```python
from build123d import *

# Parameters (mm, degrees)
SKETCH1_W                               = 16
SKETCH1_H                               = 16
BASE_DEPTH                              = 45
SKETCH3_R                               = 8
SLOTFORANOTHERPART_DEPTH                = 9
CHAMFERFORSLOT_DEPTH                    = 9
M5X0_8_TAPPED_HOLE_FOR_SLOTSCREW_D      = 4.2
M5X0_8_TAPPED_HOLE_FOR_SLOTSCREW_DEPTH  = 11.1381927
M5X0_8_TAPPED_HOLE_FOR_SLOTSCREW_TIP    = 1.2618073
M3X0_5_TAPPED_HOLE_FOR_ROD_FIXING_D     = 2.5
M3X0_5_TAPPED_HOLE_FOR_ROD_FIXING_DEPTH = 6.748924226
M3X0_5_TAPPED_HOLE_FOR_ROD_FIXING_TIP   = 0.751075774
F_10_2_10_2_ROD_HOLE_D                  = 10.2
F_10_2_10_2_ROD_HOLE_DEPTH              = 11.935610843
F_10_2_10_2_ROD_HOLE_CSINK_D            = 11
F_10_2_10_2_ROD_HOLE_CSINK_ANGLE        = 90
F_10_2_10_2_ROD_HOLE_TIP                = 3.064389157


with BuildPart() as part:
    # Sketch1 → Base (new body)
    with BuildSketch(Plane.XY):
        Rectangle(SKETCH1_W, SKETCH1_H)
    extrude(amount=BASE_DEPTH)

    # Sketch3 → SlotForAnotherPart (cut, through all)
    with BuildSketch(Plane(origin=(0, 0, 0), x_dir=(0, 0, -1), z_dir=(1, 0, 0))):
        with BuildLine():
            Line((-8.000000039, 8), (-18, 8))
            Line((-18, 8), (-18, -8))
            Line((-18, -8), (-8, -8))
            ThreePointArc((-8, -8), (-16, -1.9e-08), (-8.000000039, 8))
        make_face()
        with Locations((-8, 0)):
            Circle(SKETCH3_R)
        with BuildLine():
            Line((1.927362357, 8), (-8.000000039, 8))
            ThreePointArc((-8.000000039, 8), (-2.343145764, 5.656854263), (0, 0))
            ThreePointArc((0, 0), (-2.343145751, -5.656854249), (-8, -8))
            Line((-8, -8), (1.927362357, -8))
            Line((1.927362357, -8), (1.927362357, 8))
        make_face()
    extrude(amount=-SLOTFORANOTHERPART_DEPTH, mode=Mode.SUBTRACT)

    # Sketch3_3 → ChamferForSlot (cut, through all)
    with BuildSketch(Plane(origin=(0, 0, 0), x_dir=(0, 0, -1), z_dir=(1, 0, 0))):
        with BuildLine():
            Line((1.927362357, 8), (-8.000000039, 8))
            ThreePointArc((-8.000000039, 8), (-2.343145764, 5.656854263), (0, 0))
            ThreePointArc((0, 0), (-2.343145751, -5.656854249), (-8, -8))
            Line((-8, -8), (1.927362357, -8))
            Line((1.927362357, -8), (1.927362357, 8))
        make_face()
    extrude(amount=CHAMFERFORSLOT_DEPTH, mode=Mode.SUBTRACT)

    # M5x0.8 Tapped Hole for SlotScrew
    with Locations(Plane(origin=(8, 0, 0), x_dir=(0, 0, -1), z_dir=(1, 0, 0))):
        with Locations((-8, 0)):
            Hole(M5X0_8_TAPPED_HOLE_FOR_SLOTSCREW_D / 2, depth=M5X0_8_TAPPED_HOLE_FOR_SLOTSCREW_DEPTH)
            with Locations((0, 0, -(M5X0_8_TAPPED_HOLE_FOR_SLOTSCREW_DEPTH + M5X0_8_TAPPED_HOLE_FOR_SLOTSCREW_TIP / 2))):  # 118° drill point
                Cone(0, M5X0_8_TAPPED_HOLE_FOR_SLOTSCREW_D / 2, M5X0_8_TAPPED_HOLE_FOR_SLOTSCREW_TIP, mode=Mode.SUBTRACT)

    # M3x0.5 Tapped Hole for Rod Fixing
    with Locations(Plane(origin=(8, 0, 0), x_dir=(0, 0, -1), z_dir=(1, 0, 0))):
        with Locations((-40, 0)):
            Hole(M3X0_5_TAPPED_HOLE_FOR_ROD_FIXING_D / 2, depth=M3X0_5_TAPPED_HOLE_FOR_ROD_FIXING_DEPTH)
            with Locations((0, 0, -(M3X0_5_TAPPED_HOLE_FOR_ROD_FIXING_DEPTH + M3X0_5_TAPPED_HOLE_FOR_ROD_FIXING_TIP / 2))):  # 118° drill point
                Cone(0, M3X0_5_TAPPED_HOLE_FOR_ROD_FIXING_D / 2, M3X0_5_TAPPED_HOLE_FOR_ROD_FIXING_TIP, mode=Mode.SUBTRACT)

    # 10.2 _10.2_ Rod Hole
    with Locations(Plane.XY.offset(45)):
        with Locations((0, 0)):
            CounterSinkHole(F_10_2_10_2_ROD_HOLE_D / 2, F_10_2_10_2_ROD_HOLE_CSINK_D / 2, depth=F_10_2_10_2_ROD_HOLE_DEPTH, counter_sink_angle=F_10_2_10_2_ROD_HOLE_CSINK_ANGLE)
            with Locations((0, 0, -(F_10_2_10_2_ROD_HOLE_DEPTH + F_10_2_10_2_ROD_HOLE_TIP / 2))):  # 118° drill point
                Cone(0, F_10_2_10_2_ROD_HOLE_D / 2, F_10_2_10_2_ROD_HOLE_TIP, mode=Mode.SUBTRACT)


solid = part.part
```
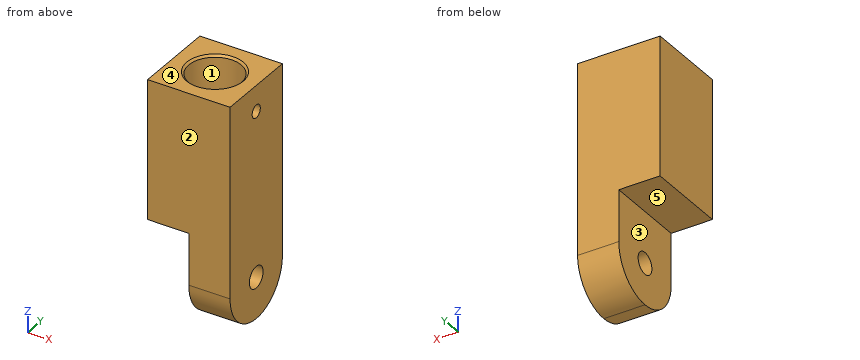
Build history of the part. All positions in model axes, mm. Face numbers are marked on the shaded views. A direction names the side the tool comes from. Coordinates: 2 decimals unless noted, no trailing zeros. Order: outer loops, then holes, each group sorted by start corner. A loop starts at its lowest first (then second) coordinate and runs counter-clockwise, first axis right, second up.
Item 1: Drop flat-ended pins along their axis: pin 1 Ø5 at (y, z) = (-2.5, 7) entering from -X; pin 2 Ø6 at (x, y) = (-5, 0) entering from -Z. Give the stop position or say it passes through.
Filled in:
pin 1: stops at x = 0
pin 2: stops at z = 18
Item 2: Tool access for the marked faces 4 and 5: list every direction of +Z, -Z, +X, -X, +Y, -Y with a clear straight run to the whole face (end or side of a thin tool).
Filled in:
face 4: +Z, +X, -X, +Y, -Y
face 5: -Z, -X, +Y, -Y
Item 3: Saw through at C-C on x = -6.25. List the corners of the cut face in (y, z).
Filled in:
outline: (-8, 18) - (8, 18) - (8, 45) - (-8, 45) - close
Item 4: Saw through at D-D on z = 13. List the corners of the cut face in (x, y).
Filled in:
outline: (0, -8) - (8, -8) - (8, 8) - (0, 8) - close
Item 5: Saw through at B-B on z = 7.5. List the corners of the cut face in (x, y).
Filled in:
outline: (0, -7.98) - (8, -7.98) - (8, -2.04) - (0, -2.04) - close; (0, 2.04) - (8, 2.04) - (8, 7.98) - (0, 7.98) - close
Item 6: Mould opens along Y. For the marked faces 1, 2 and 3 say: released by +Y, released by -Y, zero draft, split by the parting line, or undercut.
Filled in:
face 1: undercut
face 2: released by -Y
face 3: zero draft
Item 7: Saw through at A-A on z = 40. List the corners of the cut face in (x, y), then the cut area to 3 significant figures.
Filled in:
outline: (-8, -8) - (8, -8) - (8, -1.25) - (4.94, -1.25) arc R5.1 cw (long way) to (4.94, 1.25) - (8, 1.25) - (8, 8) - (-8, 8) - close
area: 167 mm2
Item 8: Drill centre lines: L1, parallel to X at y = 0, z = 37; L2, parallel to Y at x = 6.5, z = 40; L3, parallel to Z at x = -4.75, y = -3.25. Where is each one in solid material? Low to high.
Filled in:
L1: x = -8 to -5.1, 5.1 to 8
L2: y = -8 to -1.25, 1.25 to 8
L3: z = 18 to 45
